For this review, take the finished solid that the model builds, in its own axes (mm). A direction names the side the tool comes from. Coordinates: 2 decimals unless noted, no trailing zeros. Loops run counter-clockwise (first coordinate to the right, second up) from the corner with the lowest first, then second, coordinate; pieces in that order, holes last. Notation, with made-up numbers: M -16,54 L 6,54 A32 ccw 6,88 Z; hole C -4.5,-32 d5. An arc over 180 degrees is marked long. Answer as a JSON object with one key per item and string values. Group by question number.
Item 1: Add section B-B (y = 19.25). Count the separate pieces of the cut face and the enclosed holes in it, then the cut area to 3 significant figures.
Item 2: Add section A-A (y = 13.48). State the section outline as (x, z) points, then the cut area to 3 significant figures.
Item 3: Add section C-C (z = 33). State the section outline as (x, y) points.
Item 4: Insertion check: pin 1 (2 mm diameter, centred on x = 7.5, z = -3.51, fed in from +Y); pin 2 (2.5 mm diameter, centred on y = 18, z = 23, fed in from +X); pin 3 (6 mm diameter, centred on y = 14.5, z = 2, fed in from +X); pin 4 (3 mm diameter, centred on x = -3.5, z = 7.49, fed in from -Y). Each pin has a flat end and moves straight along its axis. Give the tip position at first contact, or say it passes through.
Item 5: Mouldability with a two-part tool opening along Z and no side actions: class faces 1 (the face through (-1, 19, 72.094)), 2 (the face through (-22.388, 19, 64)), 3 (the face through (6.25, 18.88, -0.07)) as +Z half, -Z half, draft (parallel to the pull), parting line (faces both ways), or undercut.
Item 6: Tool access review of faces 4 (the face through (-7, 19, 23)), 5 (the face through (-3.5, 13, 42)), 6 (the face through (0.181, 18.881, -10.526)): name each direction out of +Z, -Z, +X, -X, +Y, -Y from which nothing blocks a thin tool from reaching the whole face with its end or side.
Item 7: Add section D-D (x = -15.5). State the section outline as (y, z) points.
Item 8: Wall thickness on L1, parallel to Z at x = -5.85, y = 13.48; L2, parallel to Z at x = -8.5, y = 20; L3, parallel to Z at x = -4, y = 12: over which ranges is each line inside the solid? List them lowest first. Write a range as from..to.
from build123d import *

# Parameters (mm, degrees)
BOSS_EXTRUDE1_START     = -3
BOSS_EXTRUDE1_OUTLINE_R = 1.25
BOSS_EXTRUDE1_DEPTH     = 3
SKETCH6_W               = 3
SKETCH6_H               = 29.12999922
BOSS_EXTRUDE3_DEPTH     = 11.68
SKETCH9_R               = 1.75
CUT_EXTRUDE2_DEPTH      = 5
SKETCH10_W              = 43.550923211
SKETCH10_H              = 3
BOSS_EXTRUDE4_DEPTH     = 15
SKETCH11_W              = 7
SKETCH11_H              = 3
CUT_EXTRUDE3_DEPTH      = 10


# Read off the part's stored shape, not the designer's step: Boss-Extrude1
with BuildPart() as part:
    # Boss-Extrude1 outline → Boss-Extrude1 (new body)
    with BuildSketch(Plane(origin=(0, 0, 0), x_dir=(1, 0, 0), z_dir=(0, 1, 0)).offset(BOSS_EXTRUDE1_START)):
        with BuildLine():
            Line((21.162477615, -57.094438481), (21.162544036, -28.414715022))
            Line((21.162544036, -28.414715022), (9.924191255, 3.512841719))
            ThreePointArc((9.924191255, 3.512841719), (0, 10.527565199), (-9.924191255, 3.512841719))
            Line((-9.924191255, 3.512841719), (-22.339897891, -28.212185032))
            Line((-22.339897891, -28.212185032), (-22.388445596, -57.094438481))
            Line((-22.388445596, -57.094438481), (21.162477615, -57.094438481))
        make_face()
        with Locations((-3.499861001, -7.487216855)):
            Circle(BOSS_EXTRUDE1_OUTLINE_R, mode=Mode.SUBTRACT)
        with Locations((-7.42819985, -3.486548919)):
            Circle(BOSS_EXTRUDE1_OUTLINE_R, mode=Mode.SUBTRACT)
        with Locations((-7.499989222, 0.012714758)):
            Circle(BOSS_EXTRUDE1_OUTLINE_R, mode=Mode.SUBTRACT)
        with Locations((-7.500049059, 3.512714758)):
            Circle(BOSS_EXTRUDE1_OUTLINE_R, mode=Mode.SUBTRACT)
        with Locations((-3.500117445, 7.512783142)):
            Circle(BOSS_EXTRUDE1_OUTLINE_R, mode=Mode.SUBTRACT)
        with Locations((0.000138999, -7.487157018)):
            Circle(BOSS_EXTRUDE1_OUTLINE_R, mode=Mode.SUBTRACT)
        with Locations((3.499402676, -7.415367646)):
            Circle(BOSS_EXTRUDE1_OUTLINE_R, mode=Mode.SUBTRACT)
        with Locations((7.500070612, -3.487028797)):
            Circle(BOSS_EXTRUDE1_OUTLINE_R, mode=Mode.SUBTRACT)
        with Locations((7.500010775, 0.012971203)):
            Circle(BOSS_EXTRUDE1_OUTLINE_R, mode=Mode.SUBTRACT)
        with Locations((-0.000117446, 7.512842979)):
            Circle(BOSS_EXTRUDE1_OUTLINE_R, mode=Mode.SUBTRACT)
        with Locations((3.499882554, 7.512902816)):
            Circle(BOSS_EXTRUDE1_OUTLINE_R, mode=Mode.SUBTRACT)
        with Locations((7.500070612, 3.512971202)):
            Circle(BOSS_EXTRUDE1_OUTLINE_R, mode=Mode.SUBTRACT)
    extrude(amount=BOSS_EXTRUDE1_DEPTH)

    # Sketch6 → Boss-Extrude3 (add)
    with BuildSketch(Plane.XZ.offset(3)):
        with Locations((-5, 42.529438871)):
            Rectangle(SKETCH6_W, SKETCH6_H)
    extrude(amount=-BOSS_EXTRUDE3_DEPTH)

    # Sketch9 → Cut-Extrude2 (cut)
    with BuildSketch(Plane(origin=(-3.5, 0, 0), x_dir=(0, 0, -1), z_dir=(1, 0, 0))):
        with Locations((-37.369439261, 3.88)):
            Circle(SKETCH9_R)
        with Locations((-47.719439261, 3.88)):
            Circle(SKETCH9_R)
    extrude(amount=-CUT_EXTRUDE2_DEPTH, mode=Mode.SUBTRACT)


with BuildPart() as body_2:
    # Mirror1: mirrored copy
    add(part.part.mirror(Plane(origin=(0, 8.68, 0), x_dir=(0, 0, 1), z_dir=(0, -1, 0))))

    # Sketch10 → Boss-Extrude4 (add)
    with BuildSketch(Plane.XY.offset(57.094438481)):
        with Locations((-0.612983991, 18.86)):
            Rectangle(SKETCH10_W, SKETCH10_H)
    extrude(amount=BOSS_EXTRUDE4_DEPTH)

    # Sketch11 → Cut-Extrude3 (cut)
    with BuildSketch(Plane.XZ.offset(-17.36)):
        with Locations((-3.5, 23.5)):
            Rectangle(SKETCH11_W, SKETCH11_H)
    extrude(amount=-CUT_EXTRUDE3_DEPTH, mode=Mode.SUBTRACT)


solid = body_2.part
From the geometry:
{
 "1": {"separate pieces": "1", "enclosed holes": "13", "area": "2,940 mm²"},
 "2": {"outline": "M -6.5,27.96 L -3.5,27.96 L -3.5,35.62 L -6.5,35.62 Z; M -6.5,39.12 L -3.5,39.12 L -3.5,45.97 L -6.5,45.97 Z; M -6.5,49.47 L -3.5,49.47 L -3.5,57.09 L -6.5,57.09 Z", "area": "66.4 mm²"},
 "3": {"outline": "M -22.35,17.36 L -6.5,17.36 L -6.5,8.68 L -3.5,8.68 L -3.5,17.36 L 21.16,17.36 L 21.16,20.36 L -22.35,20.36 Z"},
 "4": {"pin 1": "passes through", "pin 2": "stops at x = 19.7", "pin 3": "stops at x = 12.18", "pin 4": "stops at y = 17.36"},
 "5": {"face 1": "+Z half", "face 2": "draft", "face 3": "undercut"},
 "6": {"face 4": "+Y, -Y", "face 5": "+Z, -Z, +X, -Y", "face 6": "-Z, +Y, -Y"},
 "7": {"outline": "M 17.36,10.73 L 20.36,10.73 L 20.36,72.09 L 17.36,72.09 Z"},
 "8": {"L1": "z = 27.96..35.62, 39.12..45.97, 49.47..57.09", "L2": "z = -6.21..-4.26, -2.76..-0.76, 0.74..2.84, 4.13..72.09", "L3": "z = 27.96..36.44, 38.3..46.79, 48.65..57.09"}
}
